Geometry check sheet. Reference: the model listing, model coordinates, mm. A direction names the side the tool comes from. Round coordinates to 2 decimals unless told otherwise and drop trailing zeros. Loops run counter-clockwise (first coordinate to the right, second up) from the corner with the lowest first, then second, coordinate; pieces in that order, holes last. Notation, with made-up numbers: (1.5, 18) -> (46.5, 18) arc R10 cw to (46.5, 31) -> close; hole circle Ø6 at (-21, 50). An arc over 180 degrees is marked (long way). Use a Markdown table: item, result. Add a question column.
Q1. Sectioned sample at A-A, the plane z = 10.5. Enter the section's corners in (x, y).
Q2. Release check for a two-part mould opening along X. For faces 1 (the face through (-2, -1.2, 12)), 2 (the face through (8, 0, 0)) record: released by +X, released by -X, zero draft, split by the parting line, or undercut.
Q3. Sectioned sample at B-B, the plane z = -3. Give the number of separate pieces and of enclosed holes in the cut face, then the cut area to 4 significant figures.
Q4. Gauge pin test, flat ends, axial feed: P1, Ø10, axis at x = 9.5, z = 0, coming from the +Y side; P2, Ø1.5, axis at y = 5.5, z = 1.5, coming from the -X side; P3, Ø6, axis at x = -5, y = 0.5, coming from the +Z side; P4, Ø5, axis at x = -9.5, y = 5, coming from the +Z side. Record the tip position at first contact, or that the pin passes through.
Q5. Material ranges on L1, parallel to X at y = -1, z = 0; L2, parallel to Z at x = -1.75, y = 0.5; L3, parallel to Y at x = -11.5, z = 6.5, recorded low to high.
Q6. Set-up check for faces 3 (the face through (0, -1.2, 0)), 4 (the face through (-8.35, 0, 0.6)): record each of +Z, -Z, +X, -X, +Y, -Y from which the full face is reachable in a straight line by a thin tool's end or side.
Q7. Sectioned sample at D-D, the plane y = 4.75. Enter the section's corners in (x, z).
```python
from build123d import *
from build123d.topology import SkipClean

# Parameters (mm, degrees)
SALIENTE_EXTRUIR1_DEPTH = 1
MATRIZC1_COUNT          = 2
CROQUIS2_R              = 2
SALIENTE_EXTRUIR2_DEPTH = 8
REDONDEO1_R             = 2
SALIENTE_EXTRUIR3_START = 1.2
CROQUIS3_R              = 13.5
CROQUIS3_R_2            = 12
SALIENTE_EXTRUIR3_DEPTH = 1.2
SALIENTE_EXTRUIR4_START = 1.2
CROQUIS4_R              = 2
SALIENTE_EXTRUIR4_DEPTH = 1.2


with BuildPart() as part:
    # Croquis1 → Saliente-Extruir1 (new body)
    with BuildSketch(Plane(origin=(0, 0, 0), x_dir=(1, 0, 0), z_dir=(0, 1, 0))):
        with BuildLine():
            Line((0, 13.5), (0, 12))
            ThreePointArc((0, 12), (-9.980726138, 6.662214779), (-11.082290197, -4.602482373))
            add(Edge.make_bspline(
                [(-11.082290197, -4.602482373), (-11.00840419, -3.348074009), (-9.319606871, 0.45967832), (-5.885100929, 2.140100591), (-3.256465409, 1.683534759), (-2.521994609, 0.852903354), (-1.938361352, 0.49270201)],
                knots=[0, 0, 0, 0, 0.307401752, 0.611772427, 0.741286119, 1, 1, 1, 1], degree=3))
            ThreePointArc((-1.938361352, 0.49270201), (-1.227720648, 1.578829316), (0, 2))
            Line((0, 2), (0, -2))
            ThreePointArc((0, -2), (-0.610407114, -1.904574271), (-1.162565685, -1.627403155))
            add(Edge.make_bspline(
                [(-10.085301, -6.502822752), (-10.082838156, -6.506642403), (-10.985626663, -2.087609579), (-5.366270818, 1.292290157), (-2.947582336, 0.671775941), (-1.66061048, -1.320024502), (-1.162565685, -1.627403155)],
                knots=[0, 0, 0, 0, 0.481214874, 0.664290716, 0.77922591, 1, 1, 1, 1], degree=3))
            ThreePointArc((-10.085301, -6.502822752), (-5.743088323, -10.536457493), (0, -12))
            Line((0, -12), (0, -13.5))
            ThreePointArc((0, -13.5), (-13.5, 0), (0, 13.5))
        make_face()
    saliente_extruir1 = extrude(amount=SALIENTE_EXTRUIR1_DEPTH)

    # MatrizC1: Saliente-Extruir1 ×2 about axis
    matrizc1_axis = Axis((0, 1.05, 0), (0, -1, 0))
    for i in range(1, MATRIZC1_COUNT):
        add(saliente_extruir1.rotate(matrizc1_axis, i * 360 / MATRIZC1_COUNT))

    # Croquis2 → Saliente-Extruir2 (add)
    with BuildSketch(Plane(origin=(0, 1, 0), x_dir=(1, 0, 0), z_dir=(0, 1, 0))):
        with Locations(Location((0, 0, 0), (0, 0, 54.459178385))):
            Circle(CROQUIS2_R)
    extrude(amount=SALIENTE_EXTRUIR2_DEPTH)

    # Redondeo1
    redondeo1_edges = [part.edges().sort_by_distance(p)[0] for p in [
        (-1.162565685, 9, 1.627403155),
    ]]
    fillet(redondeo1_edges, radius=REDONDEO1_R)

    # Croquis3 → Saliente-Extruir3 (add)
    with BuildSketch(Plane.XZ.offset(SALIENTE_EXTRUIR3_START)):
        with Locations(Location((0, 0, 0), (0, 0, 270))):
            Circle(CROQUIS3_R)
        with Locations(Location((0, 0, 0), (0, 0, 270))):
            Circle(CROQUIS3_R_2, mode=Mode.SUBTRACT)
    extrude(amount=-SALIENTE_EXTRUIR3_DEPTH)

    # Croquis4 → Saliente-Extruir4 (add)
    with SkipClean():  # the faces are left unmerged after this step: merging them gives an invalid solid
        with BuildSketch(Plane.XZ.offset(SALIENTE_EXTRUIR4_START)):
            with Locations(Location((0, 0, 0), (0, 0, 270))):
                Circle(CROQUIS4_R)
        extrude(amount=-SALIENTE_EXTRUIR4_DEPTH)


solid = part.part
```
Values:
| question | item | result |
|---|---|---|
| 1 | outline | (-8.49, -1.2) -> (-5.81, -1.2) -> (-5.81, 1) -> (-8.49, 1) -> close; (5.81, -1.2) -> (8.49, -1.2) -> (8.49, 1) -> (5.81, 1) -> close |
| 2 | face 1 | zero draft |
| 2 | face 2 | undercut |
| 3 | separate pieces | 3 |
| 3 | enclosed holes | 0 |
| 3 | area | 7.765 mm^2 |
| 4 | P1 | y = 1 |
| 4 | P2 | x = -1.85 |
| 4 | P3 | z = 13.35 |
| 4 | P4 | through |
| 5 | L1 | -13.5 to -12, -2 to 2, 12 to 13.5 |
| 5 | L2 | -13.39 to -11.87, -0.97 to 1.07, 11.87 to 13.39 |
| 5 | L3 | -1.2 to 1 |
| 6 | face 3 | +Z, -Z, +X, -X, -Y |
| 6 | face 4 | -Y |
| 7 | outline | circle Ø4 at (0, 0) |
